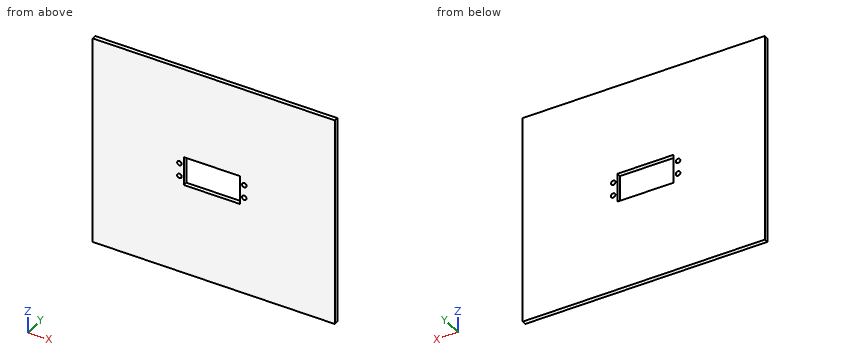
```python
from build123d import *

# Parameters (mm, degrees)
SKETCH1_W           = 184.839561026
SKETCH1_H           = 161.279122052
SKETCH1_R           = 1.75
SKETCH1_W_2         = 42.8
SKETCH1_H_2         = 22.1
BOSS_EXTRUDE1_DEPTH = 3.2


with BuildPart() as part:
    # Sketch1 → Boss-Extrude1 (new body)
    with BuildSketch(Plane(origin=(0, 0, 0), x_dir=(1, 0, 0), z_dir=(0, 1, 0))):
        with Locations((11.780219487, 0)):
            Rectangle(SKETCH1_W, SKETCH1_H)
        with Locations(Location((-14.4, 5, 0), (0, 0, 270))):
            Circle(SKETCH1_R, mode=Mode.SUBTRACT)
        with Locations(Location((-14.4, -5, 0), (0, 0, 270))):
            Circle(SKETCH1_R, mode=Mode.SUBTRACT)
        with Locations(Location((35.1, -5, 0), (0, 0, 270))):
            Circle(SKETCH1_R, mode=Mode.SUBTRACT)
        with Locations(Location((35.1, 5, 0), (0, 0, 270))):
            Circle(SKETCH1_R, mode=Mode.SUBTRACT)
        with Locations((10.35, 0)):
            Rectangle(SKETCH1_W_2, SKETCH1_H_2, mode=Mode.SUBTRACT)
    extrude(amount=-BOSS_EXTRUDE1_DEPTH)


solid = part.part
```
Can you work these out from the model? Positions are in its coordinate system, mm. Coordinates: 2 decimals unless noted, no trailing zeros. Loops run counter-clockwise (first coordinate to the right, second up) from the corner with the lowest first, then second, coordinate; pieces in that order, holes last. Notation, with made-up numbers: (49.5, -27) - (74.5, -27) arc R13 cw to (74.5, -16) - close; hole circle Ø6 at (-1, 41.25). An arc over 180 degrees is marked (long way). Answer as CSV lines item,"result". Start each with the question number.
1) Suppose I cut it at B-B (y = -1.8). Please give me the cut outline in (x, z), plus the area to 3 significant figures.
2) For pin 1 (5 mm diameter, centred on x = 37, z = 22, fed in from +Y), with a flat end and sliding along its axis, tell me the tip position at first contact or that it passes through.
3) I need wall thicknesses on line 1 (X direction, y = -1.75, z = 5); line 2 (X direction, y = -1, z = 1). Which ranges of each line are inside material? Lowest first, please. Write a range as from..to.
4) Suppose I cut it at A-A (x = 21.5). Please give me the cut outline in (y, z), plus the area to 3 significant figures.
Check result:
1,outline,"(-80.64, -80.64) - (104.2, -80.64) - (104.2, 80.64) - (-80.64, 80.64) - close; hole circle Ø3.5 at (-14.4, -5); hole circle Ø3.5 at (-14.4, 5); hole (-11.05, -11.05) - (31.75, -11.05) - (31.75, 11.05) - (-11.05, 11.05) - close; hole circle Ø3.5 at (35.1, -5); hole circle Ø3.5 at (35.1, 5)"
1,area,"28,800 mm²"
2,pin 1,"stops at y = 0"
3,line 1,"x = -80.64..-16.15, -12.65..-11.05, 31.75..33.35, 36.85..104.2"
3,line 2,"x = -80.64..-11.05, 31.75..104.2"
4,outline,"(-3.2, -80.64) - (0, -80.64) - (0, -11.05) - (-3.2, -11.05) - close; (-3.2, 11.05) - (0, 11.05) - (0, 80.64) - (-3.2, 80.64) - close"
4,area,"445 mm²"
